```python
from build123d import *

# Parameters (mm, degrees)
F0_R        = 2.5
F1_DEPTH    = 3
F2_T1_DEPTH = 3


# Not quite as in the source:
# - a fillet or chamfer that OpenCascade refuses, or shapes differently, is made with other operations: its cross-section is extruded or revolved along the edge and cut away or added


with BuildPart() as f1:
    # F0 (on Front) → F1 (new body)
    with BuildSketch(Plane.XZ):
        with BuildLine():
            Line((-85.7558696013, 2.2170336112), (-85.7558696013, -11.7829663888))
            Line((-85.7558696013, -11.7829663888), (-85.7558696013, -26.7829663888))
            ThreePointArc((-85.7558696013, -26.7829663888), (-84.2914035073, -30.3185002947), (-80.7558696013, -31.7829663888))
            Line((-80.7558696013, -31.7829663888), (-70.7558696013, -31.7829663888))
            Line((-70.7558696013, -31.7829663888), (53.2441303987, -31.7829663888))
            Line((53.2441303987, -31.7829663888), (63.2441303987, -31.7829663888))
            ThreePointArc((63.2441303987, -31.7829663888), (66.7796643046, -30.3185002947), (68.2441303987, -26.7829663888))
            Line((68.2441303987, -26.7829663888), (68.2441303987, -17.7829663888))
            Line((68.2441303987, -17.7829663888), (68.2441303987, -11.7829663888))
            Line((68.2441303987, -11.7829663888), (68.2441303987, -2.7829663888))
            Line((68.2441303987, -2.7829663888), (68.2441303987, 2.2170336112))
            Line((68.2441303987, 2.2170336112), (68.2441303987, 32.2170336112))
            Line((68.2441303987, 32.2170336112), (68.2441303987, 47.2170336112))
            ThreePointArc((68.2441303987, 47.2170336112), (66.7796643046, 50.7525675171), (63.2441303987, 52.2170336112))
            Line((63.2441303987, 52.2170336112), (53.2441303987, 52.2170336112))
            Line((53.2441303987, 52.2170336112), (-70.7558696013, 52.2170336112))
            Line((-70.7558696013, 52.2170336112), (-80.7558696013, 52.2170336112))
            ThreePointArc((-80.7558696013, 52.2170336112), (-84.2914035073, 50.7525675171), (-85.7558696013, 47.2170336112))
            Line((-85.7558696013, 47.2170336112), (-85.7558696013, 32.2170336112))
            Line((-85.7558696013, 32.2170336112), (-85.7558696013, 2.2170336112))
        make_face()
        with Locations((-75.7558696013, -21.7829663888)):
            Circle(F0_R, mode=Mode.SUBTRACT)
        with BuildLine():
            ThreePointArc((-44.7558696013, 42.7170336112), (-47.2307433355, 48.6919073454), (-41.2558696013, 46.2170336112))
            Line((-41.2558696013, 46.2170336112), (23.7441303987, 46.2170336112))
            ThreePointArc((23.7441303987, 46.2170336112), (27.2441303987, 49.7170336112), (30.7441303987, 46.2170336112))
            ThreePointArc((30.7441303987, 46.2170336112), (29.7190041328, 43.7421598771), (27.2441303987, 42.7170336112))
            Line((27.2441303987, 42.7170336112), (27.2441303987, -22.2829663888))
            ThreePointArc((27.2441303987, -22.2829663888), (29.7190041328, -23.3080926546), (30.7441303987, -25.7829663888))
            ThreePointArc((30.7441303987, -25.7829663888), (27.2441303987, -29.2829663888), (23.7441303987, -25.7829663888))
            Line((23.7441303987, -25.7829663888), (-41.2558696013, -25.7829663888))
            ThreePointArc((-41.2558696013, -25.7829663888), (-47.2307433355, -28.2578401229), (-44.7558696013, -22.2829663888))
            Line((-44.7558696013, -22.2829663888), (-44.7558696013, 42.7170336112))
        make_face(mode=Mode.SUBTRACT)
        with Locations((58.2441303987, -21.7829663888)):
            Circle(F0_R, mode=Mode.SUBTRACT)
        with Locations((-75.7558696013, 42.2170336112)):
            Circle(F0_R, mode=Mode.SUBTRACT)
        with Locations((58.2441303987, 42.2170336112)):
            Circle(F0_R, mode=Mode.SUBTRACT)
        with BuildLine():
            ThreePointArc((-44.7558696013, 44.2170336112), (-46.1700831637, 47.6312471736), (-42.7558696013, 46.2170336112))
            Line((-42.7558696013, 46.2170336112), (-41.2558696013, 46.2170336112))
            ThreePointArc((-41.2558696013, 46.2170336112), (-47.2307433355, 48.6919073454), (-44.7558696013, 42.7170336112))
            Line((-44.7558696013, 42.7170336112), (-44.7558696013, 44.2170336112))
        make_face()
        with BuildLine():
            Line((-41.2558696013, 46.2170336112), (-42.7558696013, 46.2170336112))
            ThreePointArc((-42.7558696013, 46.2170336112), (-43.341656039, 44.8028200488), (-44.7558696013, 44.2170336112))
            Line((-44.7558696013, 44.2170336112), (-44.7558696013, 42.7170336112))
            ThreePointArc((-44.7558696013, 42.7170336112), (-42.2809958672, 43.7421598771), (-41.2558696013, 46.2170336112))
        make_face()
        with BuildLine():
            Line((-44.7558696013, -23.7829663888), (-44.7558696013, -22.2829663888))
            ThreePointArc((-44.7558696013, -22.2829663888), (-47.2307433355, -28.2578401229), (-41.2558696013, -25.7829663888))
            Line((-41.2558696013, -25.7829663888), (-42.7558696013, -25.7829663888))
            ThreePointArc((-42.7558696013, -25.7829663888), (-46.1700831637, -27.1971799512), (-44.7558696013, -23.7829663888))
        make_face()
        with BuildLine():
            ThreePointArc((-41.2558696013, -25.7829663888), (-42.2809958672, -23.3080926546), (-44.7558696013, -22.2829663888))
            Line((-44.7558696013, -22.2829663888), (-44.7558696013, -23.7829663888))
            ThreePointArc((-44.7558696013, -23.7829663888), (-43.341656039, -24.3687528264), (-42.7558696013, -25.7829663888))
            Line((-42.7558696013, -25.7829663888), (-41.2558696013, -25.7829663888))
        make_face()
        with BuildLine():
            Line((27.2441303987, -23.7829663888), (27.2441303987, -22.2829663888))
            ThreePointArc((27.2441303987, -22.2829663888), (24.7692566645, -23.3080926546), (23.7441303987, -25.7829663888))
            Line((23.7441303987, -25.7829663888), (25.2441303987, -25.7829663888))
            ThreePointArc((25.2441303987, -25.7829663888), (25.8299168363, -24.3687528264), (27.2441303987, -23.7829663888))
        make_face()
        with BuildLine():
            ThreePointArc((30.7441303987, -25.7829663888), (29.7190041328, -23.3080926546), (27.2441303987, -22.2829663888))
            Line((27.2441303987, -22.2829663888), (27.2441303987, -23.7829663888))
            ThreePointArc((27.2441303987, -23.7829663888), (28.658343961, -24.3687528264), (29.2441303987, -25.7829663888))
            ThreePointArc((29.2441303987, -25.7829663888), (27.2441303987, -27.7829663888), (25.2441303987, -25.7829663888))
            Line((25.2441303987, -25.7829663888), (23.7441303987, -25.7829663888))
            ThreePointArc((23.7441303987, -25.7829663888), (27.2441303987, -29.2829663888), (30.7441303987, -25.7829663888))
        make_face()
        with BuildLine():
            Line((25.2441303987, 46.2170336112), (23.7441303987, 46.2170336112))
            ThreePointArc((23.7441303987, 46.2170336112), (24.7692566645, 43.7421598771), (27.2441303987, 42.7170336112))
            Line((27.2441303987, 42.7170336112), (27.2441303987, 44.2170336112))
            ThreePointArc((27.2441303987, 44.2170336112), (25.8299168363, 44.8028200488), (25.2441303987, 46.2170336112))
        make_face()
        with BuildLine():
            ThreePointArc((30.7441303987, 46.2170336112), (27.2441303987, 49.7170336112), (23.7441303987, 46.2170336112))
            Line((23.7441303987, 46.2170336112), (25.2441303987, 46.2170336112))
            ThreePointArc((25.2441303987, 46.2170336112), (27.2441303987, 48.2170336112), (29.2441303987, 46.2170336112))
            ThreePointArc((29.2441303987, 46.2170336112), (28.658343961, 44.8028200488), (27.2441303987, 44.2170336112))
            Line((27.2441303987, 44.2170336112), (27.2441303987, 42.7170336112))
            ThreePointArc((27.2441303987, 42.7170336112), (29.7190041328, 43.7421598771), (30.7441303987, 46.2170336112))
        make_face()
    extrude(amount=F1_DEPTH)

    # F2: fillet of radius 10 on 8 edges, made by hand

    # F2_s2 → F2_t1 (join)
    with BuildSketch(Plane.XZ):
        with BuildLine():
            ThreePointArc((24.6515378061, 43.8657650921), (26.5734946341, 40.7482665367), (27.2441303987, 37.1478550376))
            Line((27.2441303987, 37.1478550376), (27.2441303987, 42.7170336112))
            ThreePointArc((27.2441303987, 42.7170336112), (25.8262869335, 43.0170773758), (24.6515378061, 43.8657650921))
        make_face()
        with BuildLine():
            ThreePointArc((18.1749518251, 46.2170336112), (21.7753633242, 45.5463978466), (24.8928618796, 43.6244410186))
            ThreePointArc((24.8928618796, 43.6244410186), (24.0441741633, 44.7991901461), (23.7441303987, 46.2170336112))
            Line((23.7441303987, 46.2170336112), (18.1749518251, 46.2170336112))
        make_face()
        with BuildLine():
            ThreePointArc((-42.4046010823, 43.6244410186), (-39.2871025268, 45.5463978466), (-35.6866910277, 46.2170336112))
            Line((-35.6866910277, 46.2170336112), (-41.2558696013, 46.2170336112))
            ThreePointArc((-41.2558696013, 46.2170336112), (-41.5559133659, 44.7991901461), (-42.4046010823, 43.6244410186))
        make_face()
        with BuildLine():
            ThreePointArc((-42.1632770087, 43.8657650921), (-44.0852338368, 40.7482665367), (-44.7558696013, 37.1478550376))
            Line((-44.7558696013, 37.1478550376), (-44.7558696013, 42.7170336112))
            ThreePointArc((-44.7558696013, 42.7170336112), (-43.3380261362, 43.0170773758), (-42.1632770087, 43.8657650921))
        make_face()
        with BuildLine():
            ThreePointArc((-42.1632770087, -23.4316978697), (-44.0852338368, -20.3141993143), (-44.7558696013, -16.7137878152))
            Line((-44.7558696013, -16.7137878152), (-44.7558696013, -22.2829663888))
            ThreePointArc((-44.7558696013, -22.2829663888), (-43.3380261362, -22.5830101534), (-42.1632770087, -23.4316978697))
        make_face()
        with BuildLine():
            ThreePointArc((-35.6866910277, -25.7829663888), (-39.2871025268, -25.1123306242), (-42.4046010823, -23.1903737962))
            ThreePointArc((-42.4046010823, -23.1903737962), (-41.5559133659, -24.3651229237), (-41.2558696013, -25.7829663888))
            Line((-41.2558696013, -25.7829663888), (-35.6866910277, -25.7829663888))
        make_face()
        with BuildLine():
            ThreePointArc((27.2441303987, -16.7137878152), (26.5734946341, -20.3141993143), (24.6515378061, -23.4316978697))
            ThreePointArc((24.6515378061, -23.4316978697), (25.8262869335, -22.5830101534), (27.2441303987, -22.2829663888))
            Line((27.2441303987, -22.2829663888), (27.2441303987, -16.7137878152))
        make_face()
        with BuildLine():
            ThreePointArc((24.8928618796, -23.1903737962), (21.7753633242, -25.1123306242), (18.1749518251, -25.7829663888))
            Line((18.1749518251, -25.7829663888), (23.7441303987, -25.7829663888))
            ThreePointArc((23.7441303987, -25.7829663888), (24.0441741633, -24.3651229237), (24.8928618796, -23.1903737962))
        make_face()
    extrude(amount=F2_T1_DEPTH)


solid = f1.part
```
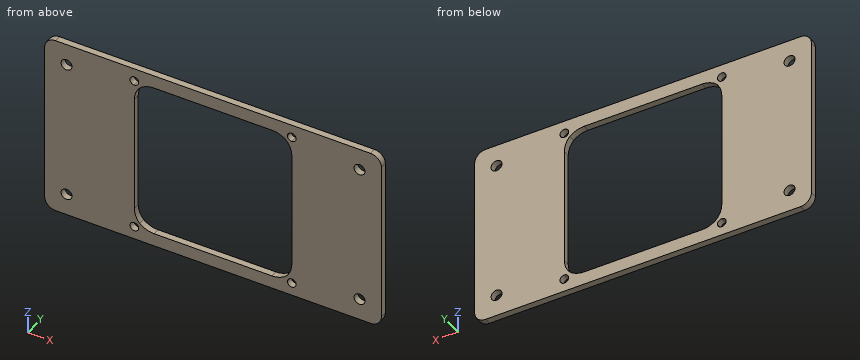
Check sheet for the modelled part. Datum: model origin and axes. Units: mm. Coordinates: 2 decimals unless noted, no trailing zeros. Order: outer loops, then holes, each group sorted by start corner. A loop starts at its lowest first (then second) coordinate and runs counter-clockwise, first axis right, second up. Notation, with made-up numbers: (79, -27) -> (90, -27) arc R28 ccw to (90, -8) -> close; hole circle Ø3 at (1.5, 8). An arc over 180 degrees is marked (long way). Write item = value, one per line. Start each with the question number.
1) Cross-section at C-C (y = -1.85). State how many separate pieces and enclosed holes the cut face has, then the cut area to 3 significant figures.
2) Cross-section at D-D (x = -76). Enter the section's corners in (y, z).
3) Cross-section at B-B (x = -26). Enter the section's corners in (y, z), then the cut area to 3 significant figures.
4) Cross-section at A-A (z = -6). Enter the section's corners in (x, y), then the cut area to 3 significant figures.
5) Material ranges on L1, parallel to X at y = -0.85, z = 34; L2, parallel to X at y = -2.5, z = 40; L3, parallel to Z at x = 7, y = -2.1, recorded low to high.
6) Go/stop test with a flat-tipped pin: P1, Ø3.5, axis at x = -44.76, z = 46.22, coming from the -Y side. Record where the tip stops, or that it passes through.
Ans:
q1.separate_pieces = 1
q1.enclosed_holes = 9
q1.area = 7,670 mm²
q2.outline = (-3, -31.78) -> (0, -31.78) -> (0, -24.27) -> (-3, -24.27) -> close; (-3, -19.29) -> (0, -19.29) -> (0, 39.73) -> (-3, 39.73) -> close; (-3, 44.71) -> (0, 44.71) -> (0, 52.22) -> (-3, 52.22) -> close
q3.outline = (-3, -31.78) -> (0, -31.78) -> (0, -25.78) -> (-3, -25.78) -> close; (-3, 46.22) -> (0, 46.22) -> (0, 52.22) -> (-3, 52.22) -> close
q3.area = 36.0 mm²
q4.outline = (-85.76, -3) -> (-44.76, -3) -> (-44.76, 0) -> (-85.76, 0) -> close; (27.24, -3) -> (68.24, -3) -> (68.24, 0) -> (27.24, 0) -> close
q4.area = 246 mm²
q5.L1 = -85.76 to -44.76, 27.24 to 68.24
q5.L2 = -85.76 to -76.91, -74.6 to -44.34, 26.83 to 57.09, 59.4 to 68.24
q5.L3 = -31.78 to -25.78, 46.22 to 52.22
q6.P1 = through
